Study the drawing (mm; zero at the part's minimum x, y, z) and answer. A direction names the side the tool comes from. Give positions to 0.01 mm unless a question says otherwise; leave off trailing zeros. Order: outer loops, then holes, each group sorted by start corner. A loop starts at its lowest first (then second) coordinate and runs counter-clockwise, first axis right, second up. Notation, with made-up numbers: (50, 29) - (90, 29) arc R8 cw to (90, 39) - close; hole circle Ø10 at (28, 63.25). An arc over 180 degrees is marked (long way). Return JSON: item names as keys, results as strings.
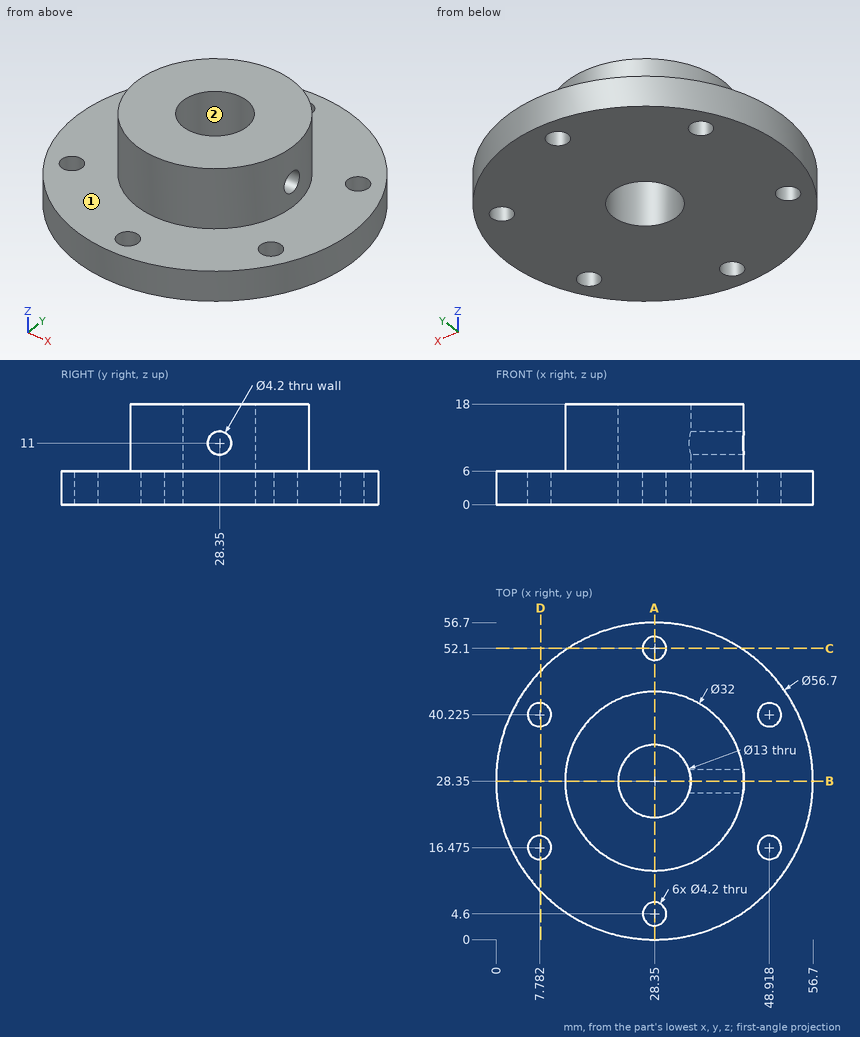
Q1. A cutting plane is placed at D-D (x = 8). Write down the section's boundary in (y, z), and give its area (3 significant figures).
Values:
{"outline": "(8.61, 0) - (14.39, 0) - (14.39, 6) - (8.61, 6) - close; (18.56, 0) - (38.14, 0) - (38.14, 6) - (18.56, 6) - close; (42.31, 0) - (48.09, 0) - (48.09, 6) - (42.31, 6) - close", "area": "187 mm²"}
Q2. For the marked faces 1 and 2, determine the directions among +Z, -Z, +X, -X, +Y, -Y from which every point of the face is accessible in a straight line to the end or side of a thin tool.
Values:
{"face 1": "+Z", "face 2": "+Z, -Z"}
Q3. A cutting plane is placed at C-C (y = 52.1). Write down the section's boundary in (x, z).
Values:
{"outline": "(12.87, 0) - (26.25, 0) - (26.25, 6) - (12.87, 6) - close; (30.45, 0) - (43.83, 0) - (43.83, 6) - (30.45, 6) - close"}
Q4. Consider L1, parallel to Y at x = 28.35, z = 4.5; L2, parallel to Z at x = 38.5, y = 28.5; L3, parallel to X at y = 38.5, z = 3.5 (1 decimal). Determine where each line is inside the solid, lowest interval first.
Values:
{"L1": "y = 0 to 2.5, 6.7 to 21.85, 34.85 to 50, 54.2 to 56.7", "L2": "z = 0 to 8.91, 13.09 to 18", "L3": "x = 1.9 to 6.6, 9 to 47.7, 50.1 to 54.8"}
Q5. A cutting plane is placed at A-A (x = 28.35). Write down the section's boundary in (y, z), and give its area (3 significant figures).
Values:
{"outline": "(0, 0) - (2.5, 0) - (2.5, 6) - (0, 6) - close; (6.7, 0) - (21.85, 0) - (21.85, 18) - (12.35, 18) - (12.35, 6) - (6.7, 6) - close; (34.85, 0) - (50, 0) - (50, 6) - (44.35, 6) - (44.35, 18) - (34.85, 18) - close; (54.2, 0) - (56.7, 0) - (56.7, 6) - (54.2, 6) - close", "area": "440 mm²"}
Q6. Given pin 1 (2 mm diameter, centred on x = 19.5, z = 11, fed in from -Y); pin 2 (5.5 mm diameter, centred on x = 48.92, y = 16.47, fed in from +Z); pin 3 (10 mm diameter, centred on x = 7, z = 4.5, fed in from -Y), each flat-ended and moving along its own axis, determine where each tip first touches the part or whether it passes through.
Values:
{"pin 1": "stops at y = 14.41", "pin 2": "stops at z = 6", "pin 3": "stops at y = 5.19"}
Q7. A cutting plane is placed at B-B (y = 28.35). Write down the section's boundary in (x, z), and give its area (3 significant figures).
Values:
{"outline": "(0, 0) - (21.85, 0) - (21.85, 18) - (12.35, 18) - (12.35, 6) - (0, 6) - close; (34.85, 0) - (56.7, 0) - (56.7, 6) - (44.35, 6) - (44.35, 8.9) - (34.85, 8.9) - close; (34.85, 13.1) - (44.35, 13.1) - (44.35, 18) - (34.85, 18) - close", "area": "450 mm²"}
